Autodesk Inventor part; units mm, degrees
ref_plane "YZ Plane" through (0, 0, 0) normal (1, 0, 0) x (0, 1, 0)
ref_plane "XZ Plane" through (0, 0, 0) normal (0, 1, 0) x (-1, 0, 0)
ref_plane "XY Plane" through (0, 0, 0) normal (0, 0, 1) x (1, 0, 0)
sketch "Sketch1" plane through (0, 0, 0) normal (1, 0, 0) x (0, 1, 0)
  line L0 (0, 0) -> (21.5526, 21.5526)
  line L1 (21.5526, 21.5526) -> (49.3914, -6.2862)
  line L2 (0, -98.8011) -> (0, 41.6267)
  line L3 (49.3914, -6.2862) -> (0, -55.6776)
  line L4 (0, 0) -> (0, -55.6776)
  line L5 (26.9408, 16.1645) -> (0, -10.7763) construction
  dimension "d0" = 39.37
  dimension "d1" = 45
  dimension "d5" = 7.62
  dimension "d6" = 38.1
extrude "Extrusion1" add sketch "Sketch1" along normal mid plane 39.37
sketch "Sketch2" plane through (-19.685, 21.5526, 21.5526) normal (0, 0.7071, 0.7071) x (1, 0, 0)
  line L0 (0, 0) -> (39.37, 0) construction
  line L1 (39.37, 0) -> (39.37, 39.37) construction
  line L2 (0, 0) -> (39.37, 39.37) construction
  line L3 (39.37, 39.37) -> (0, 39.37) construction
  line L4 (0, 39.37) -> (39.37, 0) construction
  line L5 (6.35, 6.35) -> (33.02, 6.35)
  line L6 (33.02, 6.35) -> (33.02, 33.02)
  line L7 (33.02, 33.02) -> (6.35, 33.02)
  line L8 (6.35, 33.02) -> (6.35, 6.35)
  line L9 (6.35, 6.35) -> (33.02, 33.02) construction
  line L10 (33.02, 6.35) -> (6.35, 33.02) construction
  point P0 (19.685, 0)
  point P1 (19.685, 19.685)
  dimension "d7" = 26.67
extrude "Extrusion2" cut sketch "Sketch2" against normal blind 38.1
sketch "Sketch3" plane through (0, 0, 0) normal (1, 0, 0) x (0, 1, 0)
  line L0 (21.5526, 21.5526) -> (0, 0)
  line L1 (0, 0) -> (0, -55.6776)
  line L2 (0, -55.6776) -> (49.3914, -6.2862)
  line L3 (17.9605, -28.7368) -> (0, -10.7763)
  line L4 (26.0427, 17.0625) -> (0, -8.9803)
  line L5 (0, 0) -> (0, -55.6776)
  line L6 (21.5526, 21.5526) -> (8.0019, 21.5526) construction
  line L7 (0, 0) -> (21.5526, 21.5526)
  line L8 (0, 0) -> (0, 59.6526)
  line L9 (49.3914, -6.2862) -> (0, -55.6776)
  line L10 (0, -55.6776) -> (0, -81.0776)
  line L11 (0, -136.9011) -> (0, 92.4267)
  line L12 (0, 59.6526) -> (-9.525, 59.6526)
  line L13 (-9.525, 59.6526) -> (-9.525, -81.0776)
  line L14 (-9.525, -81.0776) -> (0, -81.0776)
  point P0 (1.0999, -13.335)
  point P1 (0, -15.24)
  point P2 (0, -10.7763)
  dimension "d10" = 38.1
  dimension "d11" = 25.4
  dimension "d12" = 9.525
  dimension "supportBaseLength" = 140.7302
extrude "Extrusion3" add sketch "Sketch3" along normal mid plane 25.4
sketch "Sketch5" plane through (0, 0, 0) normal (1, 0, 0) x (0, 1, 0)
  line L0 (0, 0) -> (21.5526, 21.5526)
  line L1 (0, 59.6526) -> (0, 0)
  line L2 (21.5526, 21.5526) -> (49.3914, -6.2862)
  line L3 (21.5526, 21.5526) -> (0, 21.5526)
  line L4 (0, 0) -> (21.5526, 21.5526)
extrude "Extrusion5" add sketch "Sketch5" along normal mid plane 25.4
sketch "Sketch4" plane through (0, 0, 0) normal (0, 0, 1) x (1, 0, 0)
  line L0 (19.685, 49.3914) -> (-19.685, 49.3914)
  line L1 (19.685, 0) -> (19.685, 49.3914)
  line L2 (19.685, 0) -> (12.7, 0)
  line L3 (12.7, 0) -> (-12.7, 0)
  line L4 (-12.7, 0) -> (-19.685, 0)
  line L5 (-19.685, 49.3914) -> (-19.685, 0)
  line L6 (-12.7, 0) -> (-12.7, -9.525)
  line L7 (12.7, -9.525) -> (-12.7, -9.525)
  line L8 (12.7, -9.525) -> (12.7, 0)
  line L9 (-12.7, 0) -> (-19.685, 6.985)
  line L10 (-19.685, 49.3914) -> (-19.685, 0)
  line L11 (-19.685, 6.985) -> (-19.685, 0)
  line L12 (0, 0) -> (0, 49.3914) construction
  line L13 (12.7, 0) -> (19.685, 0)
  line L14 (12.7, 0) -> (19.685, 6.985)
  line L15 (19.685, 6.985) -> (19.685, 0)
  dimension "d15" = 45
extrude "Extrusion4" cut sketch "Sketch4" against normal up to surface (140.7302 mm away) from surface at 59.6526 contours L1 L2 L14 | L9 L4 L5
sketch "Sketch6" plane through (-12.7, 0, 59.6526) normal (0, 1, 0) x (1, 0, 0)
  line L0 (25.4, 140.7302) -> (0, 140.7302) construction
  line L1 (12.7, 140.7302) -> (12.7, 0) construction
  line L2 (25.4, 0) -> (0, 0) construction
  point P0 (12.7, 59.6526)
  point P1 (12.7, 128.0302)
  point P2 (12.7, 12.7)
  dimension "d21" = 12.7
  dimension "d22" = 12.7
hole "Hole1" at (0, 0, -68.3776) at (0, 0, 46.9526) direction (0, -1, 0) diameter 5.6134 end through all
sketch "Sketch9" plane through (0, 0, 0) normal (1, 0, 0) x (0, 1, 0)
  line L0 (0.635, -8.3453) -> (0.635, -11.4113)
  line L1 (0.635, -11.4113) -> (17.9605, -28.7368)
  line L2 (44.9013, -1.7961) -> (17.9605, -28.7368)
  line L3 (26.0427, 17.0625) -> (44.9013, -1.7961)
  line L4 (26.0427, 17.0625) -> (0.635, -8.3453)
  line L5 (35.472, 7.6332) -> (8.5312, -19.3076) construction
  line L6 (0.635, -11.4113) -> (17.9605, -28.7368) construction
  circle A0 centre (22.0016, -5.8372) radius 2.8067
  point P0 (0, 0)
  dimension "d30" = 5.6134
extrude "Extrusion6" cut sketch "Sketch9" along normal through all both and the other way through all contours A0
sketch "Sketch10" plane through (-19.685, 49.3914, -6.2862) normal (0, 0.7071, -0.7071) x (1, 0, 0)
  line L0 (6.35, 0) -> (33.02, 0) construction
  line L1 (19.685, 0) -> (19.685, 77.7875) construction
  point P0 (19.685, 30.48)
  point P1 (19.685, 19.05)
  dimension "d33" = 19.05
hole "Hole2" at (0, 35.921, -19.7566) direction (0, -0.7071, 0.7071) diameter 5.6134 depth 6.35
equation "\"d0\" = widthToSupportExtrusion"
equation "\"d1\" = attachementAngle"
equation "\"d6\" = insertDepth"
equation "\"d2\" = widthToSupportExtrusion"
equation "\"d7\" = insertForExtrusion"
equation "\"d8\" = insertDepth"
equation "\"d10\" = lenghtUnderBrace"
equation "\"d11\" = backLength"
equation "\"d12\" = supportBaseDepth"
equation "\"d13\" = supportBaseWidth"
equation "\"d19\" = supportBaseWidth"
equation "\"attachementAngle\" = 45deg"
equation "\"extrusionSize\" = 25.4"
equation "\"wallThickness\" = 6.35"
equation "\"slipClearance\" = 0.635"
equation "\"insertForExtrusion\" = extrusionSize + 2 * slipClearance"
equation "\"widthToSupportExtrusion\" = insertForExtrusion + 2 * wallThickness"
equation "\"insertDepth\" = 38.1"
equation "\"supportBaseWidth\" = 25.4"
equation "\"supportBaseDepth\" = 9.525"
equation "\"supportHoleDistanceFromEnd\" = 12.7"
equation "\"lenghtUnderBrace\" = 38.1"
equation "\"backLength\" = 25.4"
properties part number "45DegreeAttachementV03"
Build history of the part. All positions in model axes, mm. A direction names the side the tool comes from. Round coordinates to 2 decimals unless told otherwise and drop trailing zeros. Loops run counter-clockwise (first coordinate to the right, second up) from the corner with the lowest first, then second, coordinate; pieces in that order, holes last. Notation, with made-up numbers: (75.5, -2.5) -> (112.5, -2.5) arc R22 cw to (112.5, 24.5) -> close; hole circle Ø9 at (-7, 74.25). An arc over 180 degrees is marked (long way). One line per item, written item: value. Start each with the question number.
Q1. Cut at B-B on x = 5. List the corners of the cut face in (y, z) (3 decimals).
Q2. Cut at A-A on z = -67. List the corners of the cut face in (x, y) (3 decimals), plus the area to 3 significant figures.
Q3. Probe line 1 along Z through (x, y) = (0, -2.5); line 2 along Y through (x, z) = (-5, 33) (3 decimals); line 3 along Z through (x, y) = (-3, 4). List the from-to ranges inside material, lowest first.
Q4. 3-axis set-ups, long thin cutter, end or side, ignore diameter. For faces 5 (the face through (12.7, -1, -10)), 6 (the face through (0, 0, 41)), 7 (the face through (-12.7, -1, -10)), 8 (the face through (-0.19, 13.2, 4.22)), 9 (the face through (0, 0, -65)): which of +Z, -Z, +X, -X, +Y, -Y reach the whole face in a straight line?
Q5. Drop flat-ended pins along their axis: pin 1 Ø6.5 at (x, y) = (-4, 14) entering from +Z; pin 2 Ø5 at (y, z) = (-0.5, -28) entering from -X; pin 3 Ø8 at (x, z) = (-4.5, 41.5) entering from +Y. Give the stop position or say it passes through.
Q6. Cut at C-C on y = -2.5. List the corners of the cut face in (x, z).
Q7. Cut at D-D on y = 23. List the corners of the cut face in (x, z) (3 decimals).
Q8. Two-plate mould, pull along Y, no slides. Class faces 1 (the face through (2.49, 34.56, -16.56)), 2 (the face through (-0.84, -4.83, 49.63)), 3 (the face through (16.466, 19.774, -4.129)), 4 (the face through (16, 13, 13)): released by +Y, released by -Y, zero draft, split by the parting line, or undercut.
Computed:
1. outline: (-9.525, -81.078) -> (0, -81.078) -> (0, -55.678) -> (49.391, -6.286) -> (44.901, -1.796) -> (17.959, -28.738) -> (0, -10.779) -> (0, -8.98) -> (26.043, 17.062) -> (21.553, 21.553) -> (0, 21.553) -> (0, 59.653) -> (-9.525, 59.653) -> close
2. outline: (-12.7, -9.525) -> (-2.445, -9.525) -> (-2.445, 0) -> (-12.7, 0) -> close; (2.445, -9.525) -> (12.7, -9.525) -> (12.7, 0) -> (2.445, 0) -> close
2. area: 195 mm²
3. line 1: -81.08 to -71.18, -65.57 to 44.15, 49.76 to 59.65
3. line 2: -9.525 to 0
3. line 3: -51.68 to -14.78, -4.98 to 21.55
4. face 5: +Z, +X, -Y
4. face 6: +Z, +X, -X, +Y
4. face 7: +Z, -X, -Y
4. face 8: none
4. face 9: -Z, +X, -X, +Y
5. pin 1: z = 21.55
5. pin 2: x = -14.7
5. pin 3: y = 0
6. outline: (-12.7, -81.08) -> (12.7, -81.08) -> (12.7, 59.65) -> (-12.7, 59.65) -> close; hole circle Ø5.61 at (0, -68.38); hole circle Ø5.61 at (0, 46.95)
7. outline: (-19.685, -32.678) -> (19.685, -32.678) -> (19.685, -8.46) -> (13.335, -8.46) -> (13.335, -23.697) -> (-13.335, -23.697) -> (-13.335, -8.46) -> (-19.685, -8.46) -> close; (-19.685, -3.214) -> (-13.335, -3.214) -> (-13.335, 14.02) -> (13.335, 14.02) -> (13.335, -3.214) -> (19.685, -3.214) -> (19.685, 20.105) -> (-19.685, 20.105) -> close
8. face 1: undercut
8. face 2: zero draft
8. face 3: undercut
8. face 4: released by -Y
